Model file for the job. Use its own axes, mm. A direction names the side the tool comes from. Give positions to 0.01 mm unless a question says otherwise; leave off trailing zeros. Loops run counter-clockwise (first coordinate to the right, second up) from the corner with the lowest first, then second, coordinate; pieces in that order, holes last. Notation, with made-up numbers: (60, -7.75) - (101, -7.75) arc R18 ccw to (101, 20.25) - close; hole circle Ø8 at (11, 76). An arc over 180 degrees is marked (long way). Answer as CSV lines item,"result". Start each with the question number.
Item 1: Saw through at A-A on x = 0. Give the cut face in (y, z) (1 decimal), plus the area to 3 significant figures.
Item 2: Saw through at D-D on x = 42. Give the cut face in (y, z).
Item 3: Pull direction Y, two halves, no side cores. Call faces 1 (the flat face through (-1, -40, -5)), 2 (the cylindrical face through (-56.99, 62.15, -4.93)), 3 (the flat face through (-1, -20, -6.5)): pulls with the +Y half, pulls with the -Y half, needs draft (parallel to the pull), parting line crosses it, or undercut.
Item 4: Saw through at B-B on z = -2.75. State how many separate pieces and enclosed holes the cut face has, plus the area to 3 significant figures.
Item 5: Drill centre lines: L1, parallel to Y at x = 0, z = -8.85; L2, parallel to X at y = 15, z = -5.25; L3, parallel to Y at x = 0, z = -9.1. Where is each one in solid material? Low to high. Write a range as from..to.
Item 6: Tool access for faces 4 (the flat face through (-1, 13, -10)), 5 (the cylindrical face through (0.169, 62.474, -3.204)): list every direction of +Z, -Z, +X, -X, +Y, -Y with a clear straight run to the whole face (end or side of a thin tool).
Item 7: Pin check, flat tips, straight feed: pin 1 (7.5 mm diameter, centred on x = 5.5, y = -5, fed in from +Z); pin 2 (1.8 mm diameter, centred on x = 48, y = 15, fed in from -Z). Stop position of each tip, or through.
Item 8: Saw through at C-C on y = -24.25. Give the cut face in (x, z), plus the area to 3 significant figures.
from build123d import *

# Parameters (mm, degrees)
PAD_DEPTH       = 10
SKETCH_R        = 1.5
SKETCH_R_2      = 5
SKETCH_R_3      = 4
POCKET_DEPTH    = 10.001
POCKET001_DEPTH = 6.5
SKETCH006_R     = 19
SKETCH006_R_2   = 12.5
POCKET002_DEPTH = 9
SHAPEBINDER_R   = 1.5
POCKET003_DEPTH = 10.001


with BuildPart() as part:
    # Clone2D → Pad (new body)
    with BuildSketch(Plane.XY):
        with BuildLine():
            Line((-50, -40), (50, -40))
            ThreePointArc((50, -40), (57.071068, -37.071068), (60, -30))
            Line((60, -30), (60, 55))
            ThreePointArc((60, 55), (57.071068, 62.071068), (50, 65))
            Line((50, 65), (-50, 65))
            ThreePointArc((-50, 65), (-57.071068, 62.071068), (-60, 55))
            Line((-60, 55), (-60, -30))
            ThreePointArc((-60, -30), (-57.071068, -37.071068), (-50, -40))
        make_face()
    extrude(amount=-PAD_DEPTH)

    # Sketch → Pocket (cut, through all)
    with BuildSketch(Plane.XY):
        with Locations((-42.002232, -24.25)):
            Circle(SKETCH_R)
        with Locations((42.002232, -24.25)):
            Circle(SKETCH_R)
        with Locations((0, 48.5)):
            Circle(SKETCH_R_2)
        Circle(SKETCH_R_3)
    extrude(amount=-POCKET_DEPTH, mode=Mode.SUBTRACT)

    # Clone2D002 → Pocket001 (cut)
    with BuildSketch(Plane.XY):
        with BuildLine():
            ThreePointArc((10.002593, 56.7), (0, 62.475), (-10.002593, 56.7))
            Line((-10.002593, 56.7), (-54.104937, -19.6875))
            ThreePointArc((-54.104937, -19.6875), (-54.104937, -31.2375), (-44.102344, -37.0125))
            Line((-44.102344, -37.0125), (44.102344, -37.0125))
            ThreePointArc((44.102344, -37.0125), (54.104937, -31.2375), (54.104937, -19.6875))
            Line((54.104937, -19.6875), (10.002593, 56.7))
        make_face()
    extrude(amount=-POCKET001_DEPTH, mode=Mode.SUBTRACT)

    # Sketch006 → Pocket002 (cut)
    with BuildSketch(Plane.XY):
        Circle(SKETCH006_R)
        Circle(SKETCH006_R_2, mode=Mode.SUBTRACT)
    extrude(amount=-POCKET002_DEPTH, mode=Mode.SUBTRACT)

    # ShapeBinder → Pocket003 (cut, through all)
    with BuildSketch(Plane(origin=(0, 15, 0), x_dir=(0, 1, 0), z_dir=(0, 0, 1))):
        with Locations((0, 48)):
            Circle(SHAPEBINDER_R)
        with Locations((0, -48)):
            Circle(SHAPEBINDER_R)
    extrude(amount=-POCKET003_DEPTH, mode=Mode.SUBTRACT)


solid = part.part
Responses:
1,outline,"(-40, -10) - (-4, -10) - (-4, -6.5) - (-12.5, -6.5) - (-12.5, -9) - (-19, -9) - (-19, -6.5) - (-37, -6.5) - (-37, 0) - (-40, 0) - close; (4, -10) - (43.5, -10) - (43.5, -6.5) - (19, -6.5) - (19, -9) - (12.5, -9) - (12.5, -6.5) - (4, -6.5) - close; (53.5, -10) - (65, -10) - (65, 0) - (62.5, 0) - (62.5, -6.5) - (53.5, -6.5) - close"
1,area,"308 mm2"
2,outline,"(-40, -10) - (-25.75, -10) - (-25.75, -6.5) - (-37.01, -6.5) - (-37.01, 0) - (-40, 0) - close; (-22.75, -10) - (65, -10) - (65, 0) - (1.28, 0) - (1.28, -6.5) - (-22.75, -6.5) - close"
3,face 1,"pulls with the -Y half"
3,face 2,"pulls with the +Y half"
3,face 3,"undercut"
4,separate pieces,"1"
4,enclosed holes,"3"
4,area,"5,660 mm2"
5,L1,"-40..-19, -12.5..-4, 4..12.5, 19..43.5, 53.5..65"
5,L2,"-60..-49.5, -46.5..-34.08, 34.08..46.5, 49.5..60"
5,L3,"-40..-4, 4..43.5, 53.5..65"
6,face 4,"-Z, +X, -X, +Y, -Y"
6,face 5,"+Z"
7,pin 1,"z = -6.5"
7,pin 2,"through"
8,outline,"(-60, -10) - (-43.5, -10) - (-43.5, -6.5) - (-55.59, -6.5) - (-55.59, 0) - (-60, 0) - close; (-40.5, -10) - (40.5, -10) - (40.5, -6.5) - (-40.5, -6.5) - close; (43.5, -10) - (60, -10) - (60, 0) - (55.59, 0) - (55.59, -6.5) - (43.5, -6.5) - close"
8,area,"456 mm2"
